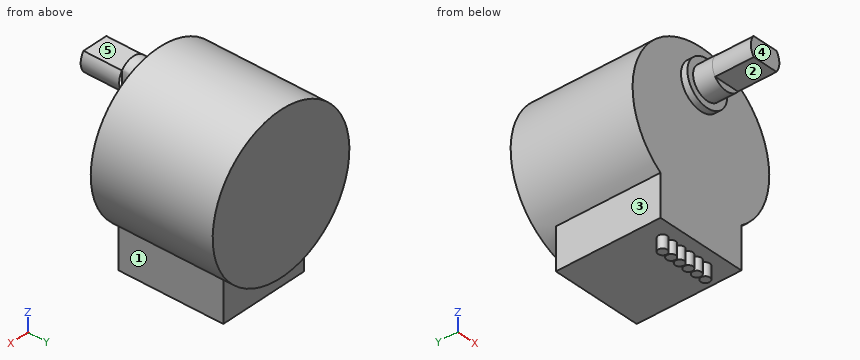
```python
from build123d import *
from build123d.topology import SkipClean

# Parameters (mm, degrees)
SKETCH_1_R      = 12
EXTRUDE_1_DEPTH = 19
SKETCH_2_W      = 14.2
SKETCH_2_H      = 6.425807527
EXTRUDE_2_DEPTH = 16.3
SKETCH_3_R      = 3.5
EXTRUDE_3_DEPTH = 1
SKETCH_4_R      = 2.5
EXTRUDE_4_DEPTH = 3
EXTRUDE_5_DEPTH = 6
SKETCH_6_R      = 0.7
EXTRUDE_6_DEPTH = 2


with BuildPart() as part:
    # 草图1 → 凸台-拉伸1 (new body)
    with BuildSketch(Plane(origin=(0, 0, 0), x_dir=(1, 0, 0), z_dir=(0, 1, 0))):
        with Locations(Location((0, 0, 0), (0, 0, 270))):
            Circle(SKETCH_1_R)
    extrude(amount=EXTRUDE_1_DEPTH)

    # 草图2 → 凸台-拉伸2 (add)
    with BuildSketch(Plane.XZ):
        with Locations((0, -12.887096236)):
            Rectangle(SKETCH_2_W, SKETCH_2_H)
    extrude(amount=-EXTRUDE_2_DEPTH)

    # 草图3 → 凸台-拉伸3 (add)
    with BuildSketch(Plane.XZ):
        with Locations(Location((0, 6.35, 0), (0, 0, 90))):
            Circle(SKETCH_3_R)
    extrude(amount=EXTRUDE_3_DEPTH)

    # 草图4 → 凸台-拉伸4 (add)
    with BuildSketch(Plane.XZ.offset(1)):
        with Locations(Location((0, 6.35, 0), (0, 0, 270))):
            Circle(SKETCH_4_R)
    extrude(amount=EXTRUDE_4_DEPTH)

    # 草图5 → 凸台-拉伸5 (add)
    with SkipClean():  # the faces are left unmerged after this step: merging them gives an invalid solid
        with BuildSketch(Plane.XZ.offset(4)):
            with BuildLine():
                Line((-2, 7.85), (2, 7.85))
                ThreePointArc((2, 7.85), (2.5, 6.35), (2, 4.85))
                Line((2, 4.85), (-2, 4.85))
                ThreePointArc((-2, 4.85), (-2.5, 6.35), (-2, 7.85))
            make_face()
        extrude(amount=EXTRUDE_5_DEPTH)

    # 草图6 → 凸台-拉伸6 (add)
    with SkipClean():  # the faces are left unmerged after this step: merging them gives an invalid solid
        with BuildSketch(Plane(origin=(0, 0, -16.1), x_dir=(-1, 0, 0), z_dir=(0, 0, -1))):
            with Locations((-3.6, 2.5)):
                Circle(SKETCH_6_R)
            with Locations((-2.1, 2.5)):
                Circle(SKETCH_6_R)
            with Locations((-0.6, 2.5)):
                Circle(SKETCH_6_R)
            with Locations((0.9, 2.5)):
                Circle(SKETCH_6_R)
            with Locations((2.4, 2.5)):
                Circle(SKETCH_6_R)
            with Locations((3.9, 2.5)):
                Circle(SKETCH_6_R)
        extrude(amount=EXTRUDE_6_DEPTH)


solid = part.part
```
For this review, take the finished solid that the model builds, in its own axes (mm). Face numbers are marked on the shaded views. A direction names the side the tool comes from. Coordinates: 2 decimals unless noted, no trailing zeros. Loops run counter-clockwise (first coordinate to the right, second up) from the corner with the lowest first, then second, coordinate; pieces in that order, holes last.
1. Add section C-C, the plane y = 12.25. Give the boundary of the cut face in (x, z), then the cut area to 3 significant figures.
2. Add section D-D, the plane x = -0.9. Give the boundary of the cut face in (y, z).
3. Add section A-A, the plane x = -3.9. Give the boundary of the cut face in (y, z).
4. Add section B-B, the plane z = -11.5. Give the boundary of the cut face in (x, y).
5. Insertion check: P1, Ø12, axis at x = 6.5, y = 9.5, coming from the -Z side; P2, Ø2, axis at x = -0.5, y = -8.5, coming from the -Z side; P3, Ø1.5, axis at x = -3.5, z = 7.5, coming from the -Y side. Each pin has a flat end and moves straight along its axis. Give the tip position at first contact, or say it passes through.
6. For the marked faces 1, 2, 3, 4 and 5, list the 3-axis set-ups (+Z, -Z, +X, -X, +Y, -Y) from which the entire face can be reached by the end or side of a thin tool; tool diameter is ignored.
7. For line 1 (Y direction, x = 1.5, z = -1.5); line 2 (X direction, y = 3.5, z = -12); line 3 (Y direction, x = -2.5, z = -12.5), list the stretches that pass through material, from the lowest coordinate up.
Result:
1. outline: (-7.1, -16.1) - (7.1, -16.1) - (7.1, -9.67) arc R12 ccw (long way) to (-7.1, -9.67) - close
1. area: 521 mm2
2. outline: (-10, 4.85) - (-4, 4.85) - (-4, 4.02) - (-1, 4.02) - (-1, 2.97) - (0, 2.97) - (0, -16.1) - (1.8, -16.1) - (1.8, -18.1) - (3.2, -18.1) - (3.2, -16.1) - (16.3, -16.1) - (16.3, -11.97) - (19, -11.97) - (19, 11.97) - (0, 11.97) - (0, 9.73) - (-1, 9.73) - (-1, 8.68) - (-4, 8.68) - (-4, 7.85) - (-10, 7.85) - close
3. outline: (0, -16.1) - (1.8, -16.1) - (1.8, -18.1) - (3.2, -18.1) - (3.2, -16.1) - (16.3, -16.1) - (16.3, -11.35) - (19, -11.35) - (19, 11.35) - (0, 11.35) - close
4. outline: (-7.1, 0) - (7.1, 0) - (7.1, 16.3) - (3.43, 16.3) - (3.43, 19) - (-3.43, 19) - (-3.43, 16.3) - (-7.1, 16.3) - close
5. P1: stops at z = -16.1
5. P2: stops at z = 4.85
5. P3: stops at y = -1
6. face 1: -Z, +X, +Y, -Y
6. face 2: -Z, +X, -X, -Y
6. face 3: -Z, -X, +Y, -Y
6. face 4: +Z, -Z, +X, -X, -Y
6. face 5: +Z, +X, -X, -Y
7. line 1: y = 0 to 19
7. line 2: x = -7.1 to 7.1
7. line 3: y = 0 to 16.3
